```python
from build123d import *

# Parameters (mm, degrees)
BOSS_EXTRU_1_DEPTH      = 10
ESQUISSE4_R             = 1.5
ENL_V_MAT_EXTRU_3_DEPTH = 10
ESQUISSE2_R             = 2
ENL_V_MAT_EXTRU_4_DEPTH = 50


with BuildPart() as part:
    # Esquisse1 → Boss.-Extru.1 (new body)
    with BuildSketch(Plane.XY):
        Polygon((-13.347674419, 16.395348837), (-3.347674419, 16.395348837), (-3.347674419, 26.395348837), (-3.347674419, 29.395348837), (16.652325581, 26.395348837), (16.652325581, 16.395348837), (26.652325581, 16.395348837), (26.652325581, -23.604651163), (-13.347674419, -23.604651163), align=None)
    extrude(amount=BOSS_EXTRU_1_DEPTH)

    # Esquisse4 → Enlèv. mat.-Extru.3 (cut)
    with BuildSketch(Plane(origin=(4.238610906, 28.257406039, 0), x_dir=(0.988936353, -0.148340453, 0), z_dir=(0.148340453, 0.988936353, 0))):
        with Locations((-4.171156291, -5.047200532)):
            Circle(ESQUISSE4_R)
        with Locations((9.052592125, -5.047200532)):
            Circle(ESQUISSE4_R)
    extrude(amount=-ENL_V_MAT_EXTRU_3_DEPTH, mode=Mode.SUBTRACT)

    # Esquisse2 → Enlèv. mat.-Extru.4 (cut)
    with BuildSketch(Plane(origin=(0, 16.395348837, 0), x_dir=(1, 0, 0), z_dir=(0, 1, 0))):
        with Locations((22.652325581, -5)):
            Circle(ESQUISSE2_R)
        with Locations((-9.347674419, -5)):
            Circle(ESQUISSE2_R)
    extrude(amount=-ENL_V_MAT_EXTRU_4_DEPTH, mode=Mode.SUBTRACT)


solid = part.part
```
The model under review builds one solid part; all positions refer to its coordinate system, in mm. A direction names the side the tool comes from. Coordinates: 2 decimals unless noted, no trailing zeros. Loops run counter-clockwise (first coordinate to the right, second up) from the corner with the lowest first, then second, coordinate; pieces in that order, holes last. Notation, with made-up numbers: (-37, 76.5) -> (14, 76.5) arc R14 ccw to (14, 92.5) -> close; hole circle Ø1 at (49, 75.5). An arc over 180 degrees is marked (long way). Answer as CSV lines item,"result".
Item 1: Take a section at B-B, the plane z = 8.25. State the section outline as (x, y) points, and give its area (3 significant figures).
Results below:
outline,"(-13.35, -23.6) -> (26.65, -23.6) -> (26.65, 16.4) -> (16.65, 16.4) -> (16.65, 26.4) -> (-3.35, 29.4) -> (-3.35, 16.4) -> (-13.35, 16.4) -> close"
area,"1,830 mm2"
Item 2: Take a section at D-D, the plane y = 25.5. Count the separate pieces of the cut face and the enclosed holes in it, and give its area (3 significant figures).
Results below:
separate pieces,"1"
enclosed holes,"2"
area,"186 mm2"
Item 3: Insertion check: pin 1 (4 mm diameter, centred on y = 18.5, z = 4.5, fed in from +X); pin 2 (5 mm diameter, centred on x = 20.5, z = 5, fed in from +Y). Each pin has a flat end and moves straight along its axis. Give the tip position at first contact, or say it passes through.
Results below:
pin 1,"stops at x = 16.65"
pin 2,"stops at y = 16.4"
Item 4: Take a section at A-A, the plane y = -4.5. State the section outline as (x, z) points.
Results below:
outline,"(-13.35, 0) -> (26.65, 0) -> (26.65, 10) -> (-13.35, 10) -> close; hole circle Ø4 at (-9.35, 5); hole circle Ø4 at (22.65, 5)"
Item 5: For L1, parallel to X at y = 7, z = 5; L2, parallel to Z at x = 22.5, y = 14; L3, parallel to X at y = -9, z = 4.5, list the stretches that pass through material, from the lowest coordinate up.
Results below:
L1,"x = -13.35 to -11.35, -7.35 to 20.65, 24.65 to 26.65"
L2,"z = 0 to 3.01, 6.99 to 10"
L3,"x = -13.35 to -11.28, -7.41 to 20.72, 24.59 to 26.65"
Item 6: Take a section at C-C, the plane x = 6. State the section outline as (y, z) points, and give its area (3 significant figures).
Results below:
outline,"(-23.6, 0) -> (27.99, 0) -> (27.99, 10) -> (-23.6, 10) -> close"
area,"516 mm2"
Item 7: Draft analysis for pull direction Y (two halves, no side actions). For faces 1 (the flat face through (11.687, 17.028, 5.026)), 2 (the flat face through (-1.39, 18.99, 5.03)), 3 (the cylindrical face through (-11.346, -3.325, 4.912)), 4 (the flat face through (20, 16.395, 5)), state which applies: +Y half, -Y half, draft (parallel to the pull), parting line (faces both ways), or undercut.
Results below:
face 1,"undercut"
face 2,"undercut"
face 3,"draft"
face 4,"+Y half"
Item 8: Machinability: for faces 5 (the flat face through (16.652, 21, 5)), 6 (the flat face through (-7, 16.395, 5)), 7 (the flat face through (7, -23.605, 5)), which of the approach directions +Z, -Z, +X, -X, +Y, -Y give a long, thin tool a straight path to every point of the face, cutting with its end or side? Answer none if there is none.
Results below:
face 5,"+Z, -Z, +X, +Y"
face 6,"+Z, -Z, -X, +Y"
face 7,"+Z, -Z, +X, -X, -Y"
